For this review, take the finished solid that the model builds, in its own axes (mm). Face numbers are marked on the shaded views. A direction names the side the tool comes from. Round coordinates to 2 decimals unless told otherwise and drop trailing zeros. Loops run counter-clockwise (first coordinate to the right, second up) from the corner with the lowest first, then second, coordinate; pieces in that order, holes last. Notation, with made-up numbers: (81.5, 78) -> (86.5, 78) arc R22 cw to (86.5, 85) -> close; hole circle Ø3 at (3, 85). An arc over 180 degrees is marked (long way). One line per question, with ' | ' between items. Start each with the question number.
1. Consider section B-B (x = 36.5). Write out the cut boundary in (y, z), and give its area (3 significant figures).
2. Consider section A-A (z = 0). Write out the cut boundary in (x, y), and give its area (3 significant figures).
3. For pin 1 Ø5 at (x, z) = (2.5, 4) entering from -Y; pin 2 Ø5 at (y, z) = (4, -1.5) entering from +X; pin 3 Ø2.5 at (x, z) = (-3.5, 0) entering from +Y; pin 4 Ø4.5 at (x, z) = (20.5, 4) entering from -Y, all flat-tipped, find the tip position at first contact; note any pin that passes through.
4. Consider section D-D (y = 10.5). Write out the cut boundary in (x, z), and give its area (3 significant figures).
5. Consider section C-C (z = 4). Write out the cut boundary in (x, y).
6. Wall thickness on line 1 along X through (y, z) = (6, 0); line 2 along X through (y, z) = (10.2, -4); line 3 along X through (y, z) = (13.25, -0.75): over which ranges is each line inside the solid? List them lowest first.
7. For the marked faces 1 and 2, list the 3-axis set-ups (+Z, -Z, +X, -X, +Y, -Y) from which the entire face can be reached by the end or side of a thin tool; tool diameter is ignored.
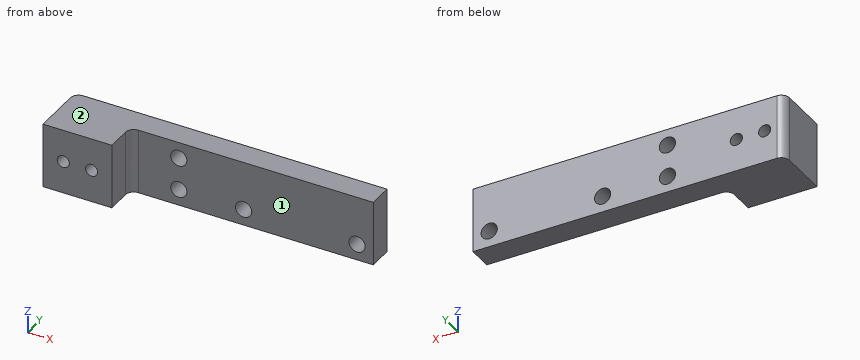
```python
from build123d import *

# Parameters (mm, degrees)
SKETCH1_W           = 17
SKETCH1_H           = 16
SKETCH1_R           = 1.5
BOSS_EXTRUDE1_DEPTH = 14
SKETCH3_W           = 16
SKETCH3_H           = 6
BOSS_EXTRUDE2_DEPTH = 60
SKETCH4_R           = 2
CUT_EXTRUDE1_DEPTH  = 71.372224634
FILLET1_R           = 2
FILLET2_R           = 2


with BuildPart() as part:
    # Sketch1 → Boss-Extrude1 (new body)
    with BuildSketch(Plane(origin=(0, 0, 0), x_dir=(1, 0, 0), z_dir=(0, 1, 0))):
        Rectangle(SKETCH1_W, SKETCH1_H)
        with Locations(Location((-3.5, 0, 0), (0, 0, 270))):
            Circle(SKETCH1_R, mode=Mode.SUBTRACT)
        with Locations(Location((3.5, 0, 0), (0, 0, 270))):
            Circle(SKETCH1_R, mode=Mode.SUBTRACT)
    extrude(amount=BOSS_EXTRUDE1_DEPTH)

    # Sketch3 → Boss-Extrude2 (add)
    with BuildSketch(Plane(origin=(8.5, 0, 0), x_dir=(0, 0, -1), z_dir=(1, 0, 0))):
        with Locations((0, 11)):
            Rectangle(SKETCH3_W, SKETCH3_H)
    extrude(amount=BOSS_EXTRUDE2_DEPTH)

    # Sketch4 → Cut-Extrude1 (cut, through all)
    with BuildSketch(Plane(origin=(0, 14, 0), x_dir=(1, 0, 0), z_dir=(0, 1, 0))):
        with Locations(Location((36.5, 4, 0), (0, 0, 270))):
            Circle(SKETCH4_R)
        with Locations(Location((64.5, 4, 0), (0, 0, 270))):
            Circle(SKETCH4_R)
        with Locations(Location((20.5, 4, 0), (0, 0, 270))):
            Circle(SKETCH4_R)
        with Locations(Location((20.5, -4, 0), (0, 0, 270))):
            Circle(SKETCH4_R)
    extrude(amount=-CUT_EXTRUDE1_DEPTH, mode=Mode.SUBTRACT)

    # Fillet1
    fillet1_edges = [part.edges().sort_by_distance(p)[0] for p in [
        (8.5, 8, 0),
    ]]
    fillet(fillet1_edges, radius=FILLET1_R)

    # Fillet2
    fillet2_edges = [part.edges().sort_by_distance(p)[0] for p in [
        (-8.5, 14, 0),
    ]]
    fillet(fillet2_edges, radius=FILLET2_R)


solid = part.part
```
Answer block:
1) outline: (8, -8) -> (14, -8) -> (14, -6) -> (8, -6) -> close; (8, -2) -> (14, -2) -> (14, 8) -> (8, 8) -> close | area: 72.0 mm2
2) outline: (-8.5, 0) -> (-5, 0) -> (-5, 14) -> (-6.5, 14) arc R2 ccw to (-8.5, 12) -> close; (-2, 0) -> (2, 0) -> (2, 14) -> (-2, 14) -> close; (5, 0) -> (8.5, 0) -> (8.5, 6) arc R2 cw to (10.5, 8) -> (68.5, 8) -> (68.5, 14) -> (5, 14) -> close | area: 514 mm2
3) pin 1: stops at y = 0 | pin 2: stops at x = 8.56 | pin 3: passes through | pin 4: stops at y = 8
4) outline: (-8.5, -8) -> (68.5, -8) -> (68.5, 8) -> (-8.5, 8) -> close; hole circle Ø3 at (-3.5, 0); hole circle Ø3 at (3.5, 0); hole circle Ø4 at (20.5, -4); hole circle Ø4 at (20.5, 4); hole circle Ø4 at (36.5, -4); hole circle Ø4 at (64.5, -4) | area: 1,170 mm2
5) outline: (-8.5, 0) -> (8.5, 0) -> (8.5, 6) arc R2 cw to (10.5, 8) -> (18.5, 8) -> (18.5, 14) -> (-6.5, 14) arc R2 ccw to (-8.5, 12) -> close; (22.5, 8) -> (68.5, 8) -> (68.5, 14) -> (22.5, 14) -> close
6) line 1: x = -8.5 to -5, -2 to 2, 5 to 8.5 | line 2: x = -8.5 to 18.5, 22.5 to 34.5, 38.5 to 62.5, 66.5 to 68.5 | line 3: x = -8.06 to -4.8, -2.2 to 2.2, 4.8 to 68.5
7) face 1: +Z, -Z, +X, -Y | face 2: +Z, +X, -X, +Y, -Y
